Here's how the part is built. I have some questions about the finished solid (model axes, mm). Give positions to 0.01 mm unless a question says otherwise; leave off trailing zeros. Loops run counter-clockwise (first coordinate to the right, second up) from the corner with the lowest first, then second, coordinate; pieces in that order, holes last.
Q1. If we section it at A-A (z = 387.5): Please give me the cut outline in (x, y).
Q2. Will these pins go through, and if not, where does the flat tip stop? P1, Ø8, axis at y = 9.5, z = 433.5, coming from the -X side; P2, Ø4, axis at x = -9.5, z = 217, coming from the +Y side; P3, Ø1, axis at x = 3.5, z = 312.5, coming from the -Y side; P4, Ø5, axis at y = 2.5, z = 343.5, coming from the -X side.
Q3. I need wall thicknesses on line 1 (X direction, y = 0, z = 356); line 2 (Y direction, x = -20.5, z = 290.5). Which ranges of each line are inside material? Lowest first, please.
Q4. We'd pull the mould along X, two halves only. Please class faces 1 (the face through (-11.434, 19.575, 498.158)), 2 (the face through (-23.12, 0.11, 24.02)), 3 (the face through (-3.141, 23.925, 251.227)): +X half, -X half, draft (parallel to the pull), parting line (faces both ways), or undercut.
from build123d import *

# Parameters (mm, degrees)
F0_R          = 24.13
F0_R_2        = 22.3012
F1_DEPTH      = 509.5875
F3_DEPTH      = 24.131
F3_DEPTH_BACK = 24.131
F6_R          = 24.13
F7_DEPTH      = 50.8
F7_DEPTH_BACK = 50.8


with BuildPart() as f1:
    # F0 (on Top) → F1 (new body)
    with BuildSketch(Plane.XY):
        Circle(F0_R)
        Circle(F0_R_2, mode=Mode.SUBTRACT)
    extrude(amount=F1_DEPTH)

    # F2 (on Right) → F3 (cut, two sides)
    with BuildSketch(Plane.YZ) as f3_sk:
        Polygon((-24.13, 48.26), (-24.13, 0), (24.13, 0), align=None)
    extrude(amount=-F3_DEPTH, mode=Mode.SUBTRACT)
    extrude(f3_sk.sketch, amount=F3_DEPTH_BACK, mode=Mode.SUBTRACT)

    # F6 (on line) → F7 (cut, two sides)
    with BuildSketch(Plane(origin=(0, 0, 0), x_dir=(0.8660254038, 0.5, 0), z_dir=(0.5, -0.8660254038, 0))) as f7_sk:
        with Locations((0, 522.2875)):
            Circle(F6_R)
    extrude(amount=-F7_DEPTH, mode=Mode.SUBTRACT)
    extrude(f7_sk.sketch, amount=F7_DEPTH_BACK, mode=Mode.SUBTRACT)


solid = f1.part
Check sheet entries:
1. outline: circle Ø48.26 at (0, 0); hole circle Ø44.6 at (0, 0)
2. P1: stops at x = -23.49
2. P2: stops at y = 22.93
2. P3: stops at y = -23.94
2. P4: stops at x = -24.13
3. line 1: x = -24.13 to -22.3, 22.3 to 24.13
3. line 2: y = -12.73 to -8.78, 8.78 to 12.73
4. face 1: undercut
4. face 2: draft
4. face 3: parting line
